Here's the drawing with two shaded views (mm, measured from the low corner). I have some questions. A direction names the side the tool comes from. Coordinates: 2 decimals unless noted, no trailing zeros. Order: outer loops, then holes, each group sorted by start corner. A loop starts at its lowest first (then second) coordinate and runs counter-clockwise, first axis right, second up. Notation, with made-up numbers: (14, 85) - (39, 85) arc R33 ccw to (39, 123) - close; hole circle Ø4 at (-27.75, 39.25). An arc over 180 degrees is marked (long way). Answer as a JSON object with one key per item and string values. Group by question number.
(1) Will this pin go through, and if not, where does the flat tip stop? P1, Ø1, axis at y = 36.5, z = 17.5, coming from the +X side (3 decimals).
(2) Which directions (+Z, -Z, +X, -X, +Y, -Y) give clear straight access to the entire face, cutting with the end or side of a thin tool? Please do the marked faces 1 and 2.
(3) Imagine slicing it at C-C, the plane z = 60. Write out the boundary of the cut face in (x, y) (3 decimals).
(4) Imagine slicing it at B-B, the plane y = 74. Write out the boundary of the cut face in (x, z) (3 decimals).
(5) Imagine slicing it at D-D, the plane x = 7.75. Write out the boundary of the cut face in (y, z) (1 decimal), and give its area (3 significant figures).
(6) Please list where these lines run through material, in increasing order: probe 1 along Z at (x, y) = (22.5, 39) (3 decimals); probe 2 along X at (y, z) = (50, 73) (3 decimals); probe 3 along Z at (x, y) = (4, 21) (1 decimal).
(7) Imagine slicing it at A-A, the plane x = 22. Write out the boundary of the cut face in (y, z) (1 decimal).
(8) We'd pull the mould along Z, two halves only. Please class the marked faces 3, 4 and 5: pulls with the +Z half, pulls with the -Z half, needs draft (parallel to the pull), parting line crosses it, or undercut.
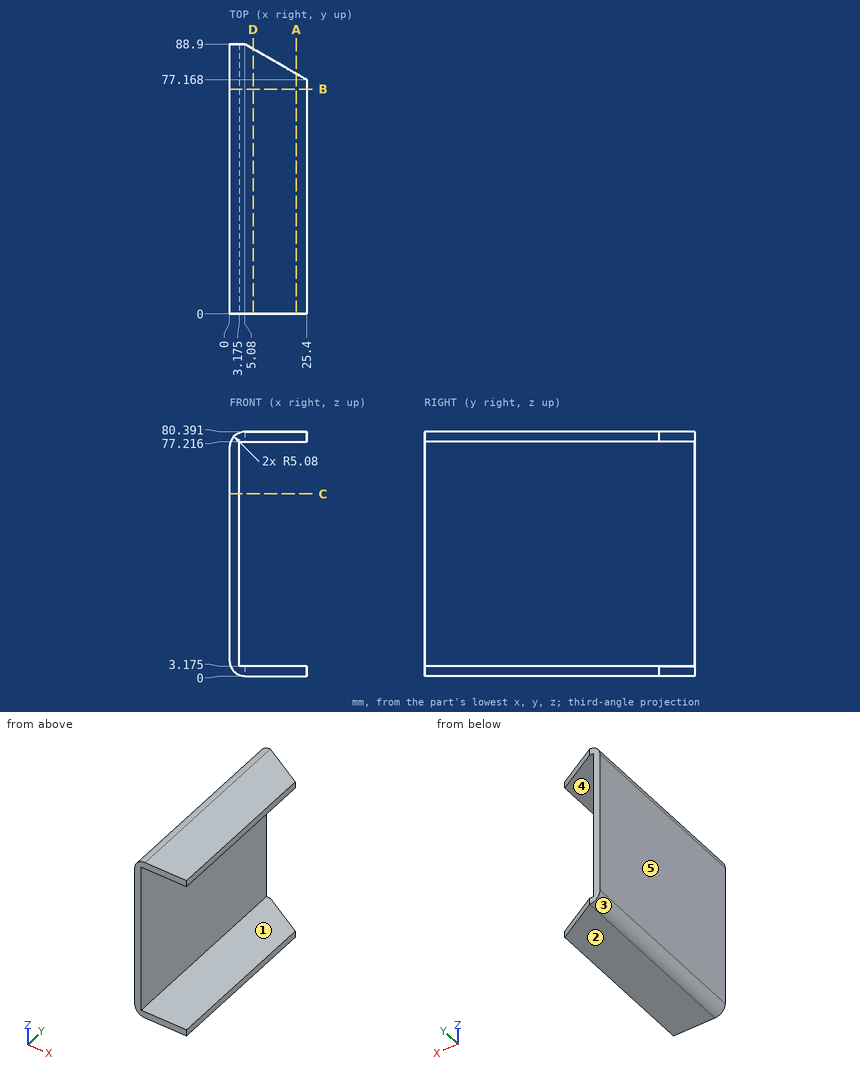
Result set:
{
 "1": {"P1": "stops at x = 3.175"},
 "2": {"face 1": "+X, +Y, -Y", "face 2": "-Z, +X, -X, +Y, -Y"},
 "3": {"outline": "(0, 0) - (3.175, 0) - (3.175, 88.9) - (0, 88.9) - close"},
 "4": {"outline": "(0, 5.08) arc R5.08 ccw to (5.08, 0) - (25.4, 0) - (25.4, 3.175) - (3.175, 3.175) - (3.175, 77.216) - (25.4, 77.216) - (25.4, 80.391) - (5.08, 80.391) arc R5.08 ccw to (0, 75.311) - close"},
 "5": {"outline": "(0, 0) - (87.4, 0) - (87.4, 3.2) - (0, 3.2) - close; (0, 77.2) - (87.4, 77.2) - (87.4, 80.4) - (0, 80.4) - close", "area": "555 mm^2"},
 "6": {"probe 1": "z = 0 to 3.175, 77.216 to 80.391", "probe 2": "x = 0 to 3.175", "probe 3": "z = 0.1 to 3.2, 77.2 to 80.3"},
 "7": {"outline": "(0, 0) - (79.1, 0) - (79.1, 3.2) - (0, 3.2) - close; (0, 77.2) - (79.1, 77.2) - (79.1, 80.4) - (0, 80.4) - close"},
 "8": {"face 3": "pulls with the -Z half", "face 4": "undercut", "face 5": "needs draft"}
}
